Autodesk Inventor part; units mm, degrees
ref_plane "YZ Plane" through (0, 0, 0) normal (1, 0, 0) x (0, 1, 0)
ref_plane "XZ Plane" through (0, 0, 0) normal (0, 1, 0) x (-1, 0, 0)
ref_plane "XY Plane" through (0, 0, 0) normal (0, 0, 1) x (1, 0, 0)
sketch "DM3D-SF, DX3D-SF_53" plane through (0, 0, 0) normal (0, 0, 1) x (1, 0, 0)
  line L0 (-5.8819, 9.2725) -> (7.0721, 9.2725)
  line L1 (7.0721, 9.2725) -> (7.0721, -3.11)
  line L2 (7.0721, -3.11) -> (5.9926, -3.11)
  line L3 (5.9926, -3.11) -> (5.6751, -2.7925)
  line L4 (5.6751, -2.7925) -> (5.6751, -1.205)
  line L5 (5.6751, -1.205) -> (-4.4849, -1.205)
  line L6 (-4.4849, -1.205) -> (-4.4849, -2.7925)
  line L7 (-4.4849, -2.7925) -> (-4.8024, -3.11)
  line L8 (-4.8024, -3.11) -> (-5.8819, -3.11)
  line L9 (-5.8819, -3.11) -> (-5.8819, 9.2725)
extrude "Extrusion1" add sketch "DM3D-SF, DX3D-SF_53" along normal blind 6.35
properties part number "DX3D-SF"
Geometry check sheet. Reference: the model listing, model coordinates, mm. A direction names the side the tool comes from. Give positions to 0.01 mm unless a question says otherwise; leave off trailing zeros. Write each loop counter-clockwise with the first axis right and the second up, starting at its lowest first coordinate (ties: lowest second). Pieces come first, ordered by that corner, then holes. Notation, with made-up numbers: M -7.75,-3.5 L 49.25,-3.5 A28 ccw 49.25,19.5 Z; hole C -31,12 d7. An arc over 180 degrees is marked long. Answer as CSV lines item,"result". Start each with the question number.
Q1. Tool access check on faces 1 (the face through (5.675, -2, 3)), 2 (the face through (1, 3, 6.35)). Record the directions out of +Z, -Z, +X, -X, +Y, -Y that give a thin tool (end or side, any length) a straight path to the whole face; none if there is none.
Q2. Go/stop test with flat-tipped pins: pin 1 (1.5 mm diameter, centred on x = 5, z = 5.5, fed in from -Y); pin 2 (2 mm diameter, centred on x = 1.5, z = 4, fed in from -Y) (3 decimals). Record where each tip stops, or that it passes through.
Q3. Material ranges on L1, parallel to X at y = -1.75, z = 4; L2, parallel to Y at x = -0.75, z = 1.5 (1 decimal); L3, parallel to Y at x = -4.75, z = 5.75, recorded low to high.
Q4. Section check A-A, the plane y = -1.75. Record the cut outline in (x, z).
Q5. Release check for a two-part mould opening along X. For faces 3 (the face through (7.072, 3, 3)), 4 (the face through (-5, -3.11, 3)), 5 (the face through (1, -1.205, 3)) record: pulls with the +X half, pulls with the -X half, needs draft (parallel to the pull), parting line crosses it, or undercut.
Q6. Section check B-B, the plane z = 1.5. Record the cut outline in (x, y) (1 decimal).
Geometry says:
1,face 1,"+Z, -Z, -Y"
1,face 2,"+Z, +X, -X, +Y, -Y"
2,pin 1,"y = -2.87"
2,pin 2,"y = -1.205"
3,L1,"-5.88 to -4.48, 5.68 to 7.07"
3,L2,"-1.2 to 9.3"
3,L3,"-3.06 to 9.27"
4,outline,"M -5.88,0 L -4.48,0 L -4.48,6.35 L -5.88,6.35 Z; M 5.68,0 L 7.07,0 L 7.07,6.35 L 5.68,6.35 Z"
5,face 3,"pulls with the +X half"
5,face 4,"needs draft"
5,face 5,"undercut"
6,outline,"M -5.9,-3.1 L -4.8,-3.1 L -4.5,-2.8 L -4.5,-1.2 L 5.7,-1.2 L 5.7,-2.8 L 6,-3.1 L 7.1,-3.1 L 7.1,9.3 L -5.9,9.3 Z"
